```python
from build123d import *

# Parameters (mm, degrees)
SKETCH_2_R      = 5.589622462
EXTRUDE_1_DEPTH = 0.4


with BuildPart() as part:
    # Эскиз1 → Повернуть1 (revolve)
    with BuildSketch(Plane.XY, mode=Mode.PRIVATE) as revolve_1_sk:
        Polygon((5.3, 0), (5.3, 8.4), (11.3, 8.4), (11.3, 6), (7.3, 6), (7.3, 0), align=None)
    revolve(revolve_1_sk.sketch.rotate(Axis((0, 0, 0), (0, 1, 0)), 90), axis=Axis((0, 0, 0), (0, 1, 0)))

    # Эскиз2 → Бобышка-Вытянуть1 (add)
    with BuildSketch(Plane(origin=(0, 8.4, 0), x_dir=(1, 0, 0), z_dir=(0, 1, 0))):
        Circle(SKETCH_2_R)
    extrude(amount=-EXTRUDE_1_DEPTH)


solid = part.part
```
Could you check a few things on this model? Use its own coordinates, in mm. A direction names the side the tool comes from. Give positions to 0.01 mm unless a question says otherwise; leave off trailing zeros. Loops run counter-clockwise (first coordinate to the right, second up) from the corner with the lowest first, then second, coordinate; pieces in that order, holes last. Notation, with made-up numbers: (73.25, 78.5) -> (85.25, 78.5) arc R10 ccw to (85.25, 92.5) -> close; hole circle Ø9 at (57, 67.25). An arc over 180 degrees is marked (long way). Put each result on its own line as item: value.
(1) Imagine slicing it at C-C on y = 3.5. Write out the boundary of the cut face in (x, z), plus the area to 3 significant figures.
Computed:
outline: circle Ø14.6 at (0, 0); hole circle Ø10.6 at (0, 0)
area: 79.2 mm^2
(2) Imagine slicing it at B-B on x = 2.5. Write out the boundary of the cut face in (y, z).
Computed:
outline: (0, -6.86) -> (6, -6.86) -> (6, -11.02) -> (8.4, -11.02) -> (8.4, 11.02) -> (6, 11.02) -> (6, 6.86) -> (0, 6.86) -> (0, 4.67) -> (8, 4.67) -> (8, -4.67) -> (0, -4.67) -> close
(3) I'm going to push flat-ended pins straight in: pin 1 Ø3 at (x, y) = (-7.5, 6) entering from -Z; pin 2 Ø4 at (y, z) = (3.5, -1) entering from +X; pin 3 Ø1.5 at (x, z) = (7, 7) entering from -Y. Where does each tip first touch, or does it pass through?
Computed:
pin 1: z = -9.58
pin 2: x = 7.3
pin 3: y = 6
(4) Please list where these lines run through material, in increasing order: probe 1 along X at (y, z) = (6.25, 0); probe 2 along X at (y, z) = (2, 0); probe 3 along Y at (x, z) = (8.5, -0.5). Write a range as [from, to].
Computed:
probe 1: [-11.3, -5.3], [5.3, 11.3]
probe 2: [-7.3, -5.3], [5.3, 7.3]
probe 3: [6, 8.4]
(5) Imagine slicing it at D-D on x = 6. Write out the boundary of the cut face in (y, z), plus the area to 3 significant figures.
Computed:
outline: (0, -4.16) -> (6, -4.16) -> (6, -9.58) -> (8.4, -9.58) -> (8.4, 9.58) -> (6, 9.58) -> (6, 4.16) -> (0, 4.16) -> close
area: 95.9 mm^2
(6) Thinking about a two-plate mould opening in Z: for faces 3 (the face through (0, 8.4, 0)), 4 (the face through (3.22, 4.06, 4.21)), 5 (the face through (-2.193, 2.958, -6.963)), which applies, pulls with the +Z half, pulls with the -Z half, needs draft (parallel to the pull), parting line crosses it, or undercut?
Computed:
face 3: needs draft
face 4: undercut
face 5: parting line crosses it
(7) For faces 1 (the face through (2.4, 6, -7.4)), 2 (the face through (-3.39, 7.18, -10.78)), which set-ups out of +Z, -Z, +X, -X, +Y, -Y let a thin tool reach every point of the face, with its end or its side?
Computed:
face 1: -Y
face 2: +Y, -Y
(8) Imagine slicing it at A-A on z = 0. Write out the boundary of the cut face in (x, y).
Computed:
outline: (-11.3, 6) -> (-7.3, 6) -> (-7.3, 0) -> (-5.3, 0) -> (-5.3, 8) -> (5.3, 8) -> (5.3, 0) -> (7.3, 0) -> (7.3, 6) -> (11.3, 6) -> (11.3, 8.4) -> (-11.3, 8.4) -> close
